from build123d import *

# Parameters (mm, degrees)
F0_R     = 10
F1_DEPTH = 25


with BuildPart() as f1:
    # F0 (on Top) → F1 (new body)
    with BuildSketch(Plane.XY):
        with BuildLine():
            ThreePointArc((-0.125005, 52.919645), (-15.611975, 38.354571), (-36.374445, 33.7821))
            ThreePointArc((-36.374445, 33.7821), (-56.934508, 24.760874), (-61.964058, 2.879321))
            ThreePointArc((-61.964058, 2.879321), (-47.191722, -24.185276), (-20.928604, -40.339624))
            ThreePointArc((-20.928604, -40.339624), (1.586671, -32.088196), (0, -8.161096))
            ThreePointArc((0, -8.161096), (-0.793901, 0.488122), (7.110988, 4.087009))
            ThreePointArc((7.110988, 4.087009), (15.789149, 4.999968), (22.49075, 10.588574))
            ThreePointArc((22.49075, 10.588574), (29.875343, 26.539907), (32.320302, 43.946786))
            ThreePointArc((32.320302, 43.946786), (19.485381, 60.683049), (-0.125005, 52.919645))
        make_face()
        with Locations((-15.179211, -21.183829)):
            Circle(F0_R, mode=Mode.SUBTRACT)
        with Locations((-37.679211, 8.816171)):
            Circle(F0_R, mode=Mode.SUBTRACT)
        with Locations((14.820789, 43.816171)):
            Circle(F0_R, mode=Mode.SUBTRACT)
    extrude(amount=F1_DEPTH)


solid = f1.part
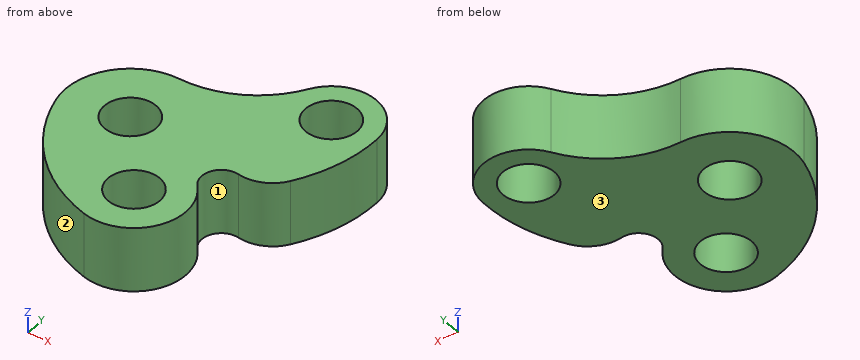
Geometry check sheet. Reference: the model listing, model coordinates, mm. Face numbers are marked on the shaded views. Give positions to 0.01 mm unless a question says otherwise; leave off trailing zeros. Order: outer loops, then holes, each group sorted by start corner. A loop starts at its lowest first (then second) coordinate and runs counter-clockwise, first axis right, second up.
1) Cross-section at D-D (y = -5). Record the boundary of the cut face in (x, z), then the cut area to 3 significant figures.
Results are:
outline: (-59.45, 0) - (-1.61, 0) - (-1.61, 25) - (-59.45, 25) - close
area: 1,450 mm2
2) Cross-section at C-C (y = -25). Record the boundary of the cut face in (x, z).
Results are:
outline: (-46.4, 0) - (-24.42, 0) - (-24.42, 25) - (-46.4, 25) - close; (-5.94, 0) - (4.45, 0) - (4.45, 25) - (-5.94, 25) - close
3) Cross-section at B-B (z = 11.25). Record the boundary of the cut face in (x, y) (3 decimals).
Results are:
outline: (-61.964, 2.879) arc R60 ccw to (-20.929, -40.34) arc R20 ccw to (0, -8.161) arc R7.5 cw to (7.111, 4.087) arc R15 ccw to (22.491, 10.589) arc R60 ccw to (32.32, 43.947) arc R17.5 ccw to (-0.125, 52.92) arc R40 cw to (-36.374, 33.782) arc R25 ccw to start; hole circle Ø20 at (-37.679, 8.816); hole circle Ø20 at (-15.179, -21.184); hole circle Ø20 at (14.821, 43.816)
4) Gauge pin test, flat ends, axial feed: pin 1 (1 mm diameter, centred on y = -20.5, z = 22, fed in from -X); pin 2 (6 mm diameter, centred on x = 6.5, y = -8, fed in from -Z); pin 3 (23 mm diameter, centred on x = 14.82, y = 43.82, fed in from -Z); pin 4 (4 mm diameter, centred on x = 10.5, z = 7, fed in from -Y). Record the tip position at first contact, or that the pin passes through.
Results are:
pin 1: stops at x = -50.81
pin 2: passes through
pin 3: stops at z = 0
pin 4: stops at y = 3.82
5) Cross-section at A-A (x = 2.5). Record the boundary of the cut face in (y, z), then the cut area to 3 significant figures.
Results are:
outline: (-30.54, 0) - (-11.83, 0) - (-11.83, 25) - (-30.54, 25) - close; (3.51, 0) - (56.24, 0) - (56.24, 25) - (3.51, 25) - close
area: 1,790 mm2
6) Material ranges on probe 1 along Y at (x, z) = (-8, 8); probe 2 along X at (y, z) = (6, 7); probe 3 along X at (y, z) = (12.5, 6.5), recorded low to high.
Results are:
probe 1: y = -39.85 to -28.15, -14.22 to 43.58
probe 2: x = -62.52 to -47.27, -28.08 to 17.74
probe 3: x = -62.41 to -46.98, -28.38 to 23.69
7) Draft check along X on the marked faces 1, 2 and 3. Enter one of: released by +X, released by -X, zero draft, split by the parting line, or undercut.
Results are:
face 1: undercut
face 2: released by -X
face 3: zero draft
